Answer from the drawing. Dimensions are ordinates in mm from the lowest x, y and z of the part. Coordinates: 2 decimals unless noted, no trailing zeros. Loops run counter-clockwise (first coordinate to the right, second up) from the corner with the lowest first, then second, coordinate; pieces in that order, holes last. Notation, with made-up numbers: (53, -13.75) - (84, -13.75) arc R19 cw to (84, 13.25) - close; hole circle Ø2 at (50.25, 35). An arc over 180 degrees is marked (long way). Write each question's results on one line, items separated by ' | '. Start each with the question number.
1. Determine the mould class of the marked faces 1, 2, 3 and 4 for opening direction Y: released by +Y, released by -Y, zero draft, split by the parting line, or undercut.
2. A cutting plane is placed at A-A on z = 26.5. Determine the outline of the cut face in (x, y), then the cut area to 3 significant figures.
3. Each of these flat-tipped pins is pushed along its axis until it touches: P1, Ø3, axis at x = 3.5, z = 18, coming from the -Y side; P2, Ø2, axis at y = 8.5, z = 17.5, coming from the -X side. Where does it stop, or does it pass through?
4. A cutting plane is placed at B-B on x = 2.5. Determine the outline of the cut face in (y, z), then the cut area to 3 significant figures.
5. Find the intervals of material crossed by line 1 along Y through (x, z) = (1.6, 25.5); line 2 along Y through (x, z) = (2.45, 3); line 3 along Z through (x, y) = (1.5, 4.25), in increasing order. Write a range as [from, to].
6. A cutting plane is placed at C-C on y = 8.5. Determine the outline of the cut face in (x, z), then the cut area to 3 significant figures.
7. A cutting plane is placed at D-D on z = 8. Determine the outline of the cut face in (x, y).
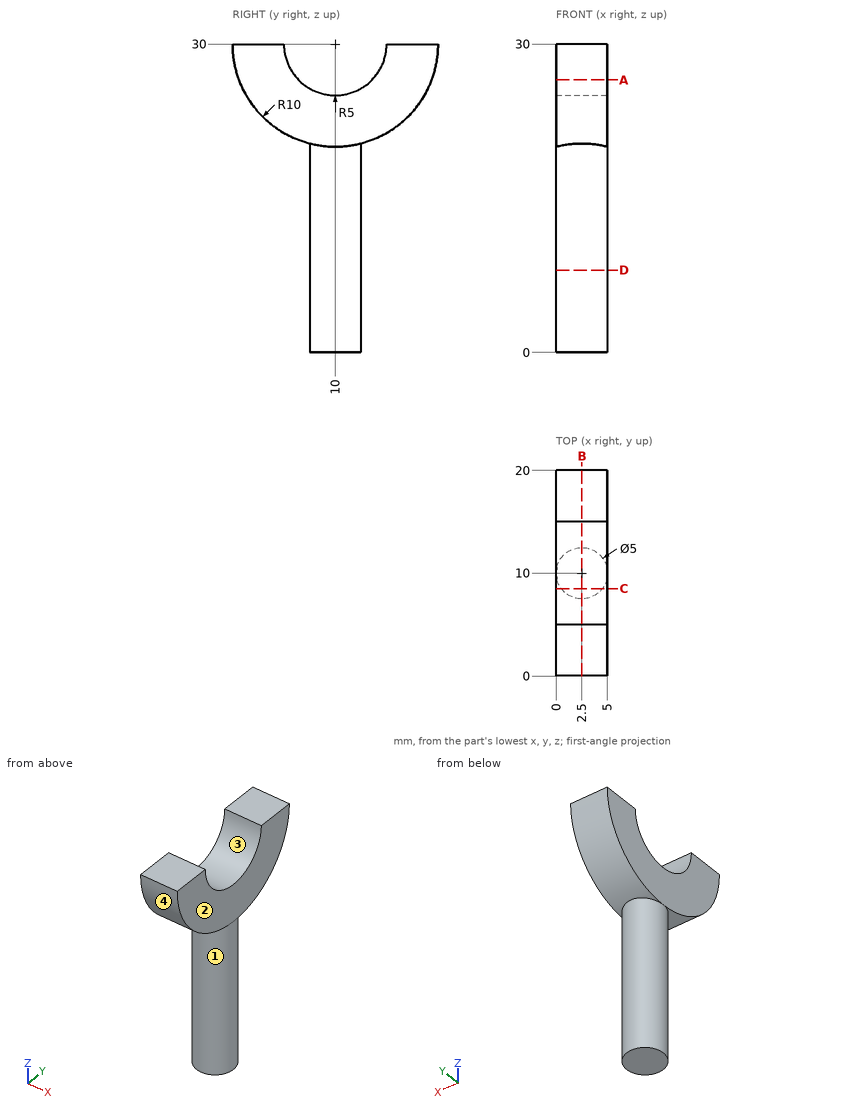
Values:
1) face 1: split by the parting line | face 2: zero draft | face 3: undercut | face 4: released by -Y
2) outline: (0, 0.63) - (5, 0.63) - (5, 6.43) - (0, 6.43) - close; (0, 13.57) - (5, 13.57) - (5, 19.37) - (0, 19.37) - close | area: 58.0 mm^2
3) P1: y = 7.5 | P2: x = 0.05
4) outline: (0, 30) arc R10 ccw to (7.5, 20.32) - (7.5, 0) - (12.5, 0) - (12.5, 20.32) arc R10 ccw to (20, 30) - (15, 30) arc R5 cw to (5, 30) - close | area: 218 mm^2
5) line 1: [1.07, 7.82], [12.18, 18.93] | line 2: [7.5, 12.5] | line 3: [21.82, 30]
6) outline: (0, 20.11) - (0.5, 20.11) - (0.5, 0) - (4.5, 0) - (4.5, 20.11) - (5, 20.11) - (5, 25.23) - (0, 25.23) - close | area: 106 mm^2
7) outline: circle Ø5 at (2.5, 10)
